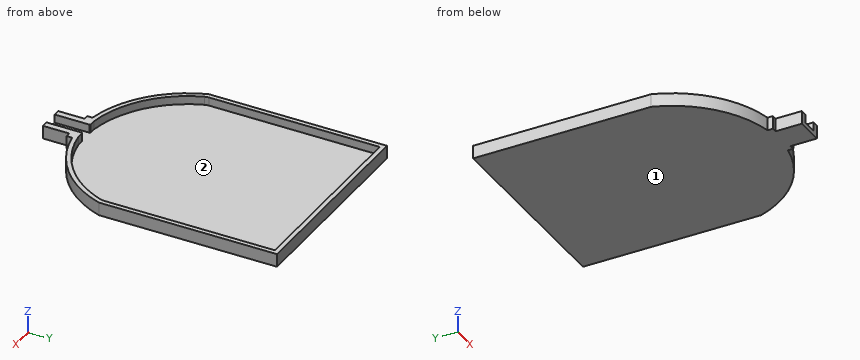
```python
from build123d import *

# Parameters (mm, degrees)
F0_W     = 5.925
F0_H     = 11.25
F0_H_2   = 1.596662
F1_DEPTH = 1
F3_DEPTH = 3.6
F4_R     = 5
F5_SIZE  = 0.25


with BuildPart() as f1:
    # F0 (on Top) → F1 (new body, symmetric)
    with BuildSketch(Plane.XY):
        with BuildLine():
            Line((2.170431, -46.027672), (-38.966179, -46.027672))
            ThreePointArc((-38.966179, -46.027672), (-23.047559, -67.17303), (2.170431, -75.209299))
            Line((2.170431, -75.209299), (2.170431, -46.027672))
        make_face()
        with BuildLine():
            ThreePointArc((2.170431, -75.209299), (27.388422, -67.17303), (43.307042, -46.027672))
            Line((43.307042, -46.027672), (2.170431, -46.027672))
            Line((2.170431, -46.027672), (2.170431, -75.209299))
        make_face()
        with BuildLine():
            Line((45.420431, 29.972328), (-41.079569, 29.972328))
            Line((-41.079569, 29.972328), (-41.079569, -46.027672))
            Line((-41.079569, -46.027672), (-38.966179, -46.027672))
            ThreePointArc((-38.966179, -46.027672), (-39.0232, -45.863777), (-39.079569, -45.699656))
            Line((-39.079569, -45.699656), (-39.079569, 27.972328))
            Line((-39.079569, 27.972328), (43.420431, 27.972328))
            Line((43.420431, 27.972328), (43.420431, -45.699656))
            ThreePointArc((43.420431, -45.699656), (43.364063, -45.863777), (43.307042, -46.027672))
            Line((43.307042, -46.027672), (45.420431, -46.027672))
            Line((45.420431, -46.027672), (45.420431, 29.972328))
        make_face()
        with BuildLine():
            Line((-38.966179, -46.027672), (-41.079569, -46.027672))
            ThreePointArc((-41.079569, -46.027672), (-27.642472, -66.108974), (-5.829569, -76.501831))
            Line((-5.829569, -76.501831), (2.170431, -76.501831))
            Line((2.170431, -76.501831), (2.170431, -75.209299))
            ThreePointArc((2.170431, -75.209299), (-23.047559, -67.17303), (-38.966179, -46.027672))
        make_face()
        with BuildLine():
            ThreePointArc((10.170431, -76.501831), (31.983335, -66.108974), (45.420431, -46.027672))
            Line((45.420431, -46.027672), (43.307042, -46.027672))
            ThreePointArc((43.307042, -46.027672), (27.388422, -67.17303), (2.170431, -75.209299))
            Line((2.170431, -75.209299), (2.170431, -76.501831))
            Line((2.170431, -76.501831), (10.170431, -76.501831))
        make_face()
        with BuildLine():
            ThreePointArc((-39.079569, -45.699656), (-39.0232, -45.863777), (-38.966179, -46.027672))
            Line((-38.966179, -46.027672), (2.170431, -46.027672))
            Line((2.170431, -46.027672), (43.307042, -46.027672))
            ThreePointArc((43.307042, -46.027672), (43.364063, -45.863777), (43.420431, -45.699656))
            Line((43.420431, -45.699656), (43.420431, 27.972328))
            Line((43.420431, 27.972328), (-39.079569, 27.972328))
            Line((-39.079569, 27.972328), (-39.079569, -45.699656))
        make_face()
        with Locations((5.132931, -84.430961)):
            Rectangle(F0_W, F0_H)
        with Locations((-0.792069, -84.430961)):
            Rectangle(F0_W, F0_H)
        with Locations((-0.792069, -78.00763)):
            Rectangle(F0_W, F0_H_2)
        with BuildLine():
            ThreePointArc((2.170431, -77.209299), (-1.845179, -77.032088), (-5.829569, -76.501831))
            Line((-5.829569, -76.501831), (-5.829569, -78.805961))
            Line((-5.829569, -78.805961), (-3.754569, -78.805961))
            Line((-3.754569, -78.805961), (-3.754569, -77.209299))
            Line((-3.754569, -77.209299), (2.170431, -77.209299))
        make_face()
        with BuildLine():
            Line((10.170431, -78.805961), (10.170431, -76.501831))
            ThreePointArc((10.170431, -76.501831), (6.186042, -77.032088), (2.170431, -77.209299))
            Line((2.170431, -77.209299), (8.095431, -77.209299))
            Line((8.095431, -77.209299), (8.095431, -78.805961))
            Line((8.095431, -78.805961), (10.170431, -78.805961))
        make_face()
        with Locations((5.132931, -78.00763)):
            Rectangle(F0_W, F0_H_2)
        with BuildLine():
            Line((2.170431, -76.501831), (-5.829569, -76.501831))
            ThreePointArc((-5.829569, -76.501831), (-1.845179, -77.032088), (2.170431, -77.209299))
            Line((2.170431, -77.209299), (2.170431, -76.501831))
        make_face()
        with BuildLine():
            ThreePointArc((2.170431, -77.209299), (6.186042, -77.032088), (10.170431, -76.501831))
            Line((10.170431, -76.501831), (2.170431, -76.501831))
            Line((2.170431, -76.501831), (2.170431, -77.209299))
        make_face()
    extrude(amount=F1_DEPTH, both=True)

    # F2 (on face) → F3 (join)
    with BuildSketch(Plane.XY.offset(1)):
        with BuildLine():
            Line((-39.079569, 27.972328), (43.420431, 27.972328))
            Line((43.420431, 27.972328), (43.420431, -45.699656))
            ThreePointArc((43.420431, -45.699656), (29.915085, -65.238213), (8.170431, -74.794342))
            Line((8.170431, -74.794342), (8.170431, -76.805961))
            Line((8.170431, -76.805961), (6.095431, -76.805961))
            Line((6.095431, -76.805961), (6.095431, -88.055961))
            Line((6.095431, -88.055961), (5.320431, -88.055961))
            Line((5.320431, -88.055961), (5.320431, -90.055961))
            Line((5.320431, -90.055961), (8.095431, -90.055961))
            Line((8.095431, -90.055961), (8.095431, -78.805961))
            Line((8.095431, -78.805961), (10.170431, -78.805961))
            Line((10.170431, -78.805961), (10.170431, -76.501831))
            ThreePointArc((10.170431, -76.501831), (31.983335, -66.108974), (45.420431, -46.027672))
            Line((45.420431, -46.027672), (45.420431, 29.972328))
            Line((45.420431, 29.972328), (-41.079569, 29.972328))
            Line((-41.079569, 29.972328), (-41.079569, -46.027672))
            ThreePointArc((-41.079569, -46.027672), (-27.642472, -66.108974), (-5.829569, -76.501831))
            Line((-5.829569, -76.501831), (-5.829569, -78.805961))
            Line((-5.829569, -78.805961), (-3.754569, -78.805961))
            Line((-3.754569, -78.805961), (-3.754569, -90.055961))
            Line((-3.754569, -90.055961), (-0.979569, -90.055961))
            Line((-0.979569, -90.055961), (-0.979569, -88.055961))
            Line((-0.979569, -88.055961), (-1.754569, -88.055961))
            Line((-1.754569, -88.055961), (-1.754569, -76.805961))
            Line((-1.754569, -76.805961), (-3.829569, -76.805961))
            Line((-3.829569, -76.805961), (-3.829569, -74.794342))
            ThreePointArc((-3.829569, -74.794342), (-25.574222, -65.238213), (-39.079569, -45.699656))
            Line((-39.079569, -45.699656), (-39.079569, 27.972328))
        make_face()
        Polygon((-0.979569, -74.794342), (-3.829569, -74.794342), (-3.829569, -76.805961), (-1.754569, -76.805961), (-1.754569, -88.055961), (-0.979569, -88.055961), align=None)
        Polygon((8.170431, -76.805961), (8.170431, -74.794342), (5.320431, -74.794342), (5.320431, -88.055961), (6.095431, -88.055961), (6.095431, -76.805961), align=None)
    extrude(amount=F3_DEPTH)

    # F4
    f4_edges = [f1.edges().sort_by_distance(p)[0] for p in [
        (-39.079569, -45.699656, 2.8),
        (43.420431, -45.699656, 2.8),
    ]]
    fillet(f4_edges, radius=F4_R)

    # F5
    f5_edges = [f1.edges().sort_by_distance(p)[0] for p in [
        (-0.979569, -74.794342, 2.8),
        (5.320431, -74.794342, 2.8),
    ]]
    chamfer(f5_edges, length=F5_SIZE)


solid = f1.part
```
Check sheet for the modelled part. Datum: model origin and axes. Units: mm. Face numbers are marked on the shaded views. Give positions to 0.01 mm unless a question says otherwise; leave off trailing zeros. Order: outer loops, then holes, each group sorted by start corner. A loop starts at its lowest first (then second) coordinate and runs counter-clockwise, first axis right, second up. Notation, with made-up numbers: M 82.25,59 L 109.25,59 A22 cw 109.25,69 Z; hole C -8.5,36.25 d9. An arc over 180 degrees is marked long. Answer in a Markdown table with one row per item.
1) Cross-section at C-C, the plane z = 2.6. Enter the section's corners in (x, y).
Filled sheet:
| item | result |
|---|---|
| outline | M -41.08,-46.03 A45.59 ccw -5.83,-76.5 L -5.83,-78.81 L -3.75,-78.81 L -3.75,-90.06 L -0.98,-90.06 L -0.98,-75.04 L -1.23,-74.79 L -3.83,-74.79 A43.59 cw -38.78,-46.56 A5 cw -39.08,-44.84 L -39.08,27.97 L 43.42,27.97 L 43.42,-44.84 A5 cw 43.12,-46.56 A43.59 cw 8.17,-74.79 L 5.57,-74.79 L 5.32,-75.04 L 5.32,-90.06 L 8.1,-90.06 L 8.1,-78.81 L 10.17,-78.81 L 10.17,-76.5 A45.59 ccw 45.42,-46.03 L 45.42,29.97 L -41.08,29.97 Z |
2) Gauge pin test, flat ends, axial feed: P1, Ø3, axis at y = -84.5, z = 3.5, coming from the -X side; P2, Ø1.7, axis at x = -5, z = 2, coming from the -Y side; P3, Ø2.5, axis at x = 9, z = 2.5, coming from the -Y side; P4, Ø3, axis at y = -83.5, z = 2.5, coming from the +X side. Record the tip position at first contact, or that the pin passes through.
Filled sheet:
| item | result |
|---|---|
| P1 | stops at x = -3.75 |
| P2 | stops at y = -78.81 |
| P3 | stops at y = -90.06 |
| P4 | stops at x = 8.1 |
3) Cross-section at A-A, the plane y = -3. Enter the section's corners in (x, z), plus the area to 3 significant figures.
Filled sheet:
| item | result |
|---|---|
| outline | M -41.08,-1 L 45.42,-1 L 45.42,4.6 L 43.42,4.6 L 43.42,1 L -39.08,1 L -39.08,4.6 L -41.08,4.6 Z |
| area | 187 mm2 |
4) Cross-section at B-B, the plane x = 12. Enter the section's corners in (y, z), plus the area to 3 significant figures.
Filled sheet:
| item | result |
|---|---|
| outline | M -76.14,-1 L 29.97,-1 L 29.97,4.6 L 27.97,4.6 L 27.97,1 L -74.09,1 L -74.09,4.6 L -76.14,4.6 Z |
| area | 227 mm2 |
5) Thickness scan on L1, parallel to X at y = -10.5, z = 3.1; L2, parallel to Z at x = 9.5, y = 15; L3, parallel to Y at x = 6, z = 3. Record the ranges inside material, lowest first. Write a range as [from, to].
Filled sheet:
| item | result |
|---|---|
| L1 | x = [-41.08, -39.08], [43.42, 45.42] |
| L2 | z = [-1, 1] |
| L3 | y = [-90.06, -74.79], [27.97, 29.97] |
6) Release check for a two-part mould opening along X. For the marked faces 1 and 2 record: +X half, -X half, draft (parallel to the pull), parting line (faces both ways), or undercut.
Filled sheet:
| item | result |
|---|---|
| face 1 | draft |
| face 2 | undercut |
